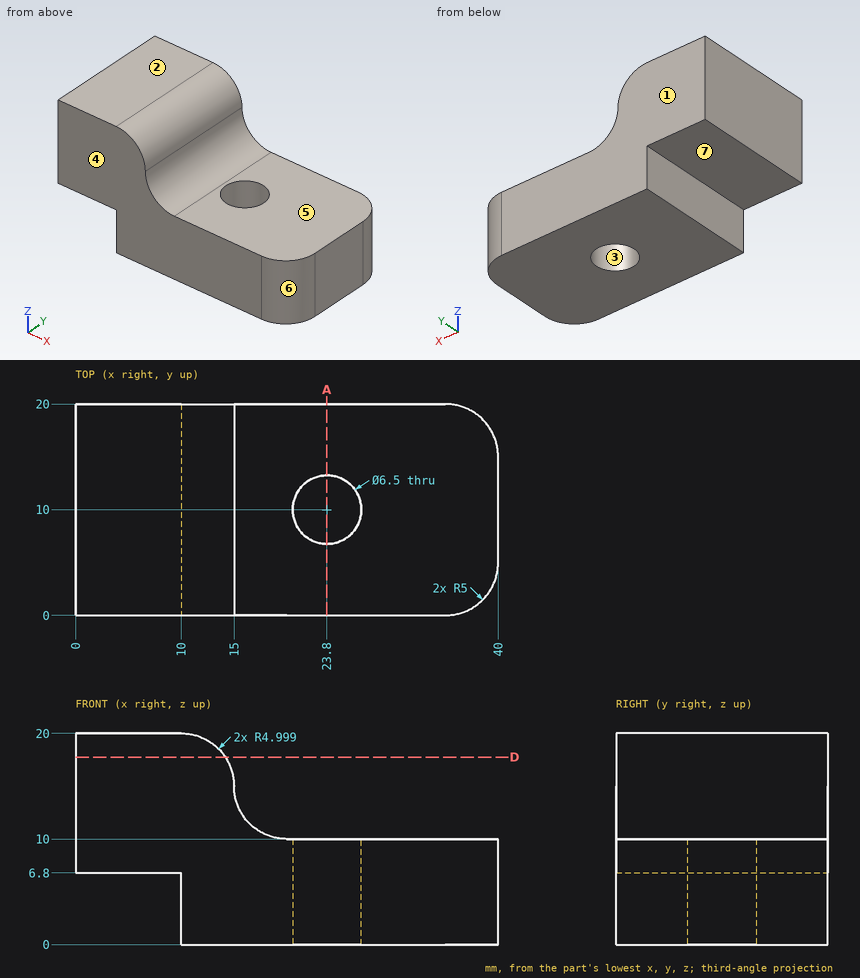
Geometry check sheet. Reference: drawing and pictorial views, mm from the part's lowest x, y, z. A direction names the side the tool comes from. Coordinates: 2 decimals unless noted, no trailing zeros. Order: outer loops, then holes, each group sorted by start corner. A loop starts at its lowest first (then second) coordinate and runs counter-clockwise, first axis right, second up. Notation, with made-up numbers: (44.25, 9) -> (54.25, 9) arc R28 ccw to (54.25, 47) -> close; hole circle Ø7 at (30, -13.5). An arc over 180 degrees is marked (long way). Use CSV: the item, a comma, the result in double quotes. Start each with the question number.
Q1. Section check D-D, the plane z = 17.75. Record the cut outline in (x, y), and give its area (3 significant figures).
Q2. Tool access check on the marked faces 5, 6 and 7. Record the directions out of +Z, -Z, +X, -X, +Y, -Y that give a thin tool (end or side, any length) a straight path to the whole face; none if there is none.
Q3. Section check A-A, the plane x = 23.8. Record the cut outline in (y, z).
Q4. Thickness scan on line 1 along X through (y, z) = (10, 4.5); line 2 along Y through (x, z) = (23.8, 4); line 3 along Z through (x, y) = (29, 12). Record the ranges inside material, lowest first.
Q5. Draft check along Y on the marked faces 1, 2, 3 and 4. Enter one of: +Y half, -Y half, draft (parallel to the pull), parting line (faces both ways), or undercut.
Q6. Depth check by flat-ended pin: P1, Ø6, axis at x = 31.5, y = 3.5, coming from the -Z side; P2, Ø10, axis at x = 27.5, y = 13, coming from the +Z side; P3, Ø7.5, axis at y = 10.5, z = 2, coming from the -X side; P4, Ø4, axis at y = 11.5, z = 13, coming from the +X side. Enter the tip coordinate at first touch or a pass-through.
Returned:
1,outline,"(0, 0) -> (14.18, 0) -> (14.18, 20) -> (0, 20) -> close"
1,area,"284 mm^2"
2,face 5,"+Z, +X, +Y, -Y"
2,face 6,"+Z, -Z, +X, -Y"
2,face 7,"-Z, -X, +Y, -Y"
3,outline,"(0, 0) -> (6.75, 0) -> (6.75, 10) -> (0, 10) -> close; (13.25, 0) -> (20, 0) -> (20, 10) -> (13.25, 10) -> close"
4,line 1,"x = 10 to 20.55, 27.05 to 40"
4,line 2,"y = 0 to 6.75, 13.25 to 20"
4,line 3,"z = 0 to 10"
5,face 1,"+Y half"
5,face 2,"draft"
5,face 3,"undercut"
5,face 4,"-Y half"
6,P1,"stops at z = 0"
6,P2,"stops at z = 10"
6,P3,"stops at x = 10"
6,P4,"stops at x = 17"
